from build123d import *

# Parameters (mm, degrees)
EXTRUDE_1_DEPTH     = 15
SKETCH_2_R          = 1.5
CUT_EXTRUDE_1_DEPTH = 20
FILLET_1_R          = 3


with BuildPart() as part:
    # 草图1 → 凸台-拉伸1 (new body)
    with BuildSketch(Plane.XY):
        Polygon((-36, 0), (36, 0), (36, -19), (51, -19), (51, -22), (33, -22), (33, -3), (-33, -3), (-33, -22), (-51, -22), (-51, -19), (-36, -19), align=None)
    extrude(amount=EXTRUDE_1_DEPTH)

    # 草图2 → 切除-拉伸1 (cut)
    with BuildSketch(Plane(origin=(0, -19, 0), x_dir=(1, 0, 0), z_dir=(0, 1, 0))):
        with Locations(Location((-43.5, -7.5, 0), (0, 0, 270))):
            Circle(SKETCH_2_R)
        with Locations(Location((43.5, -7.5, 0), (0, 0, 270))):
            Circle(SKETCH_2_R)
    extrude(amount=-CUT_EXTRUDE_1_DEPTH, mode=Mode.SUBTRACT)

    # 圆角1
    fillet_1_edges = [part.edges().sort_by_distance(p)[0] for p in [
        (-51, -20.5, 15),
        (51, -20.5, 0),
        (-51, -20.5, 0),
        (51, -20.5, 15),
    ]]
    fillet(fillet_1_edges, radius=FILLET_1_R)


solid = part.part
Input: part model. Units: mm. Frame: model coordinates. A direction names the side the tool comes from. Coordinates: 2 decimals unless noted, no trailing zeros. Write each loop counter-clockwise with the first axis right and the second up, starting at its lowest first coordinate (ties: lowest second). Pieces come first, ordered by that corner, then holes. Notation, with made-up numbers: M -1,72.5 L 12,72.5 A15 ccw 12,91.5 Z; hole C 83.5,84.5 d11. An arc over 180 degrees is marked long. Answer as a JSON object with one key per item and string values. Group by question number.
(1) Contact query for flat-ended pins moving along their axis: P1, Ø3.5, axis at x = 43.5, z = 7.5, coming from the +Y side; P2, Ø6, axis at y = -5.5, z = 3, coming from the -X side; P3, Ø7.5, axis at y = -9.5, z = 4, coming from the +X side. Output: stop coordinate, or through.
(2) Ray query, line 1 along X through (y, z) = (-20.6, 7.5); line 2 along X through (y, z) = (-11, 1.5); line 3 along Y through (x, z) = (-41.5, 1.5). Return the intervals inside material, ascending. Write a range as [from, to].
(3) Section A-A on z = 7.5. Output: boundary loops of the cut face in (x, y), plus the area to 3 significant figures.
(4) Mould query, pull axis X, two halves, no side actions, for faces 1 (the face through (-36, -10, 7)), 2 (the face through (41.7, -19, 7.4)), 3 (the face through (-33, -12, 7)), 4 (the face through (-44.964, -20.479, 7.175)). Classes: pulls with the +X half, pulls with the -X half, needs draft (parallel to the pull), parting line crosses it, or undercut.
(5) Set-up query: faces 5 (the face through (-43.6, -19, 5.7)), 6 (the face through (0.2, -2.8, 15)), 7 (the face through (33, -13, 7)). Return all of +Z, -Z, +X, -X, +Y, -Y with unobstructed straight access to the full face (end or side cutting, diameter ignored); none if empty.
(6) Section D-D on x = -32. Output: boundary loops of the cut face in (y, z), plus the area to 3 significant figures.
(7) Section C-C on x = -43.5. Output: boundary loops of the cut face in (y, z).
(8) Section B-B on y = -15. Output: boundary loops of the cut face in (x, z).
Result set:
{
 "1": {"P1": "stops at y = -19", "P2": "stops at x = -36", "P3": "stops at x = 36"},
 "2": {"line 1": "x = [-51, -45], [-42, -33], [33, 42], [45, 51]", "line 2": "x = [-36, -33], [33, 36]", "line 3": "y = [-22, -19]"},
 "3": {"outline": "M -51,-22 L -45,-22 L -45,-19 L -51,-19 Z; M -42,-22 L -33,-22 L -33,-3 L 33,-3 L 33,-22 L 42,-22 L 42,-19 L 36,-19 L 36,0 L -36,0 L -36,-19 L -42,-19 Z; M 45,-22 L 51,-22 L 51,-19 L 45,-19 Z", "area": "402 mm2"},
 "4": {"face 1": "pulls with the -X half", "face 2": "needs draft", "face 3": "undercut", "face 4": "undercut"},
 "5": {"face 5": "+Z, -Z, -X, +Y", "face 6": "+Z, +X, -X, +Y, -Y", "face 7": "+Z, -Z, -Y"},
 "6": {"outline": "M -3,0 L 0,0 L 0,15 L -3,15 Z", "area": "45.0 mm2"},
 "7": {"outline": "M -22,0 L -19,0 L -19,6 L -22,6 Z; M -22,9 L -19,9 L -19,15 L -22,15 Z"},
 "8": {"outline": "M -36,0 L -33,0 L -33,15 L -36,15 Z; M 33,0 L 36,0 L 36,15 L 33,15 Z"}
}
